Here's how the part is built. I have some questions about the finished solid (model axes, mm). A direction names the side the tool comes from. Round coordinates to 2 decimals unless told otherwise and drop trailing zeros. Write each loop counter-clockwise with the first axis right and the second up, starting at its lowest first coordinate (ties: lowest second). Pieces come first, ordered by that corner, then holes. Notation, with made-up numbers: (44.5, 34.5) - (84.5, 34.5) arc R13 ccw to (84.5, 53.5) - close; hole circle Ø2 at (50, 3). An arc over 180 degrees is marked (long way). One line per item, written item: value. Start each with the question number.
Item 1: For P1, Ø0.6, axis at y = 1, z = -10.5, coming from the -X side; P2, Ø1, axis at y = 1, z = -7, coming from the +X side; P3, Ø4, axis at x = -7.5, z = -10, coming from the +Y side; P4, Ø7, axis at x = 0, z = 0, coming from the -Y side, each with a flat end and sliding along its axis, tell me the tip position at first contact or that it passes through.
Item 2: Imagine slicing it at A-A, the plane x = 0. Please give me the cut outline in (y, z), then the cut area to 3 significant figures.
Item 3: Thinking about a two-plate mould opening in X: for faces 6 (the face through (-0.867, -0.493, 3.905)), 7 (the face through (0.1, -0.5, -27)), 8 (the face through (-10.99, -0.49, -24.15)), which applies, released by +X, released by -X, zero draft, split by the parting line, or undercut?
Item 4: Imagine slicing it at B-B, the plane z = 0. Please give me the cut outline in (x, y).
Item 5: Imagine slicing it at C-C, the plane y = 0.8. Please give me the cut outline in (x, z).
Item 6: For faces 1 (the face through (-7.934, 0.986, 6.794)), 2 (the face through (0, 1, -24.5)), 3 (the face through (-11.5, 1, -7)), 4 (the face through (8.65, 0.99, -21.49)), 5 (the face through (8.49, 0.99, 7.65)), which set-ups out of +Z, -Z, +X, -X, +Y, -Y let a thin tool reach every point of the face, with its end or its side?
Item 7: Imagine slicing it at D-D, the plane z = -13.5. Please give me the cut outline in (x, y).
Item 8: If I drill on line 1 (X direction, y = -0.55, z = 0); line 2 (Z direction, x = 0, y = -0.6); line 3 (X direction, y = 1.8, z = -2), over which ranges is the centre line in solid material (lowest first)?
```python
from build123d import *

# Parameters (mm, degrees)
BOSS_EXTRUDE1_DEPTH     = 2
BOSS_EXTRUDE3_DEPTH     = 1
SKETCH2_R               = 4
CUT_EXTRUDE1_DEPTH      = 3
CUT_EXTRUDE1_DEPTH_BACK = 2


with BuildPart() as part:
    # Sketch1 → Boss-Extrude1 (new body)
    with BuildSketch(Plane(origin=(0, 0, 0), x_dir=(1, 0, 0), z_dir=(0, 1, 0))):
        with BuildLine():
            Line((-11.5, 14.5), (-11.5, -0.5))
            ThreePointArc((-11.5, -0.5), (-8.571067812, -7.571067812), (-1.5, -10.5))
            Line((-1.5, -10.5), (1.5, -10.5))
            ThreePointArc((1.5, -10.5), (8.571067812, -7.571067812), (11.5, -0.5))
            Line((11.5, -0.5), (11.5, 14.5))
            ThreePointArc((11.5, 14.5), (8.571067812, 21.571067812), (1.5, 24.5))
            Line((1.5, 24.5), (-1.5, 24.5))
            ThreePointArc((-1.5, 24.5), (-8.571067812, 21.571067812), (-11.5, 14.5))
        make_face()
        with BuildLine():
            ThreePointArc((-1.5, 23.5), (-7.863961031, 20.863961031), (-10.5, 14.5))
            Line((-10.5, 14.5), (-10.5, -0.5))
            ThreePointArc((-10.5, -0.5), (-7.863961031, -6.863961031), (-1.5, -9.5))
            Line((-1.5, -9.5), (1.5, -9.5))
            ThreePointArc((1.5, -9.5), (7.863961031, -6.863961031), (10.5, -0.5))
            Line((10.5, -0.5), (10.5, 14.5))
            ThreePointArc((10.5, 14.5), (7.863961031, 20.863961031), (1.5, 23.5))
            Line((1.5, 23.5), (-1.5, 23.5))
        make_face(mode=Mode.SUBTRACT)
    extrude(amount=BOSS_EXTRUDE1_DEPTH)

    # Sketch1<4> → Boss-Extrude3 (add)
    with BuildSketch(Plane(origin=(0, 0, 0), x_dir=(1, 0, 0), z_dir=(0, 1, 0))):
        with BuildLine():
            Line((4, 27), (-4, 27))
            ThreePointArc((-4, 27), (-11.071067812, 24.071067812), (-14, 17))
            Line((-14, 17), (-14, -3))
            ThreePointArc((-14, -3), (-11.071067812, -10.071067812), (-4, -13))
            Line((-4, -13), (4, -13))
            ThreePointArc((4, -13), (11.071067812, -10.071067812), (14, -3))
            Line((14, -3), (14, 17))
            ThreePointArc((14, 17), (11.071067812, 24.071067812), (4, 27))
        make_face()
    extrude(amount=-BOSS_EXTRUDE3_DEPTH)

    # Sketch2 → Cut-Extrude1 (cut, two sides)
    with BuildSketch(Plane(origin=(0, 0, 0), x_dir=(1, 0, 0), z_dir=(0, 1, 0))) as cut_extrude1_sk:
        Circle(SKETCH2_R)
    extrude(amount=CUT_EXTRUDE1_DEPTH, mode=Mode.SUBTRACT)
    extrude(cut_extrude1_sk.sketch, amount=-CUT_EXTRUDE1_DEPTH_BACK, mode=Mode.SUBTRACT)


solid = part.part
```
Values follow:
1. P1: stops at x = -11.5
1. P2: stops at x = 11.5
1. P3: stops at y = 0
1. P4: passes through
2. outline: (-1, -27) - (0, -27) - (0, -24.5) - (2, -24.5) - (2, -23.5) - (0, -23.5) - (0, -4) - (-1, -4) - close; (-1, 4) - (0, 4) - (0, 9.5) - (2, 9.5) - (2, 10.5) - (0, 10.5) - (0, 13) - (-1, 13) - close
2. area: 36.0 mm^2
3. face 6: undercut
3. face 7: zero draft
3. face 8: released by -X
4. outline: (-14, -1) - (-4, -1) - (-4, 0) - (-10.5, 0) - (-10.5, 2) - (-11.5, 2) - (-11.5, 0) - (-14, 0) - close; (4, -1) - (14, -1) - (14, 0) - (11.5, 0) - (11.5, 2) - (10.5, 2) - (10.5, 0) - (4, 0) - close
5. outline: (-11.5, -14.5) arc R10 ccw to (-1.5, -24.5) - (1.5, -24.5) arc R10 ccw to (11.5, -14.5) - (11.5, 0.5) arc R10 ccw to (1.5, 10.5) - (-1.5, 10.5) arc R10 ccw to (-11.5, 0.5) - close; hole (-10.5, -14.5) arc R9 ccw to (-1.5, -23.5) - (1.5, -23.5) arc R9 ccw to (10.5, -14.5) - (10.5, 0.5) arc R9 ccw to (1.5, 9.5) - (-1.5, 9.5) arc R9 ccw to (-10.5, 0.5) - close
6. face 1: +Y
6. face 2: -Z, +X, -X, +Y
6. face 3: +Z, -Z, -X, +Y
6. face 4: -Z, +X, +Y
6. face 5: +Z, +X, +Y
7. outline: (-14, -1) - (14, -1) - (14, 0) - (11.5, 0) - (11.5, 2) - (10.5, 2) - (10.5, 0) - (-10.5, 0) - (-10.5, 2) - (-11.5, 2) - (-11.5, 0) - (-14, 0) - close
8. line 1: x = -14 to -4, 4 to 14
8. line 2: z = -27 to -4, 4 to 13
8. line 3: x = -11.5 to -10.5, 10.5 to 11.5
